```python
from build123d import *

# Parameters (mm, degrees)
CROQUIS1_R              = 0.8
CROQUIS1_R_2            = 0.5
CROQUIS1_W              = 22.5
CROQUIS1_H              = 12
SALIENTE_EXTRUIR1_DEPTH = 8
CROQUIS2_R              = 10
CORTAR_EXTRUIR1_DEPTH   = 104.387620149


with BuildPart() as part:
    # Croquis1 → Saliente-Extruir1 (new body)
    with BuildSketch(Plane.XY):
        with BuildLine():
            Line((1.5625, 24.951124098), (81.25, 19.960899278))
            ThreePointArc((81.25, 19.960899278), (100, 0), (81.25, -19.960899278))
            Line((81.25, -19.960899278), (1.5625, -24.951124098))
            ThreePointArc((1.5625, -24.951124098), (-25, 0), (1.5625, 24.951124098))
        make_face()
        Circle(CROQUIS1_R, mode=Mode.SUBTRACT)
        with Locations((66.375, 0)):
            Circle(CROQUIS1_R_2, mode=Mode.SUBTRACT)
        with Locations((93.625, 0)):
            Circle(CROQUIS1_R_2, mode=Mode.SUBTRACT)
        with Locations((7.5, 0)):
            Circle(CROQUIS1_R, mode=Mode.SUBTRACT)
        with Locations((0, -7.5)):
            Circle(CROQUIS1_R, mode=Mode.SUBTRACT)
        with Locations((-7.5, 0)):
            Circle(CROQUIS1_R, mode=Mode.SUBTRACT)
        with Locations((0, 7.5)):
            Circle(CROQUIS1_R, mode=Mode.SUBTRACT)
        with Locations((80, 0)):
            Rectangle(CROQUIS1_W, CROQUIS1_H, mode=Mode.SUBTRACT)
    extrude(amount=-SALIENTE_EXTRUIR1_DEPTH)

    # Croquis2 → Cortar-Extruir1 (cut, through all)
    with BuildSketch(Plane.XY):
        Circle(CROQUIS2_R)
    extrude(amount=-CORTAR_EXTRUIR1_DEPTH, mode=Mode.SUBTRACT)


solid = part.part
```
Model file for the job. Use its own axes, mm. A direction names the side the tool comes from. Round coordinates to 2 decimals unless told otherwise and drop trailing zeros. Write each loop counter-clockwise with the first axis right and the second up, starting at its lowest first coordinate (ties: lowest second). Pieces come first, ordered by that corner, then holes. Notation, with made-up numbers: (51.5, 60.25) -> (69.5, 60.25) arc R25 ccw to (69.5, 84.25) -> close; hole circle Ø4 at (-8.75, 86). An arc over 180 degrees is marked (long way). Answer as CSV lines item,"result".
1. Slice it at B-B, the plane z = -6.5. State how many separate pieces and enclosed holes the cut face has, plus the area to 3 significant figures.
Resolved:
separate pieces,"1"
enclosed holes,"4"
area,"4,630 mm²"
2. Pin check, flat tips, straight feed: pin 1 Ø4 at (x, z) = (76, -6) entering from +Y; pin 2 Ø2.5 at (x, z) = (84, -3.5) entering from -Y; pin 3 Ø1.5 at (x, z) = (46.5, -3) entering from -Y. Stop position of each tip, or through.
Resolved:
pin 1,"y = 20.41"
pin 2,"y = -19.81"
pin 3,"y = -22.18"
3. Slice it at A-A, the plane x = 0. List the corners of the cut face in (y, z), plus the area to 3 significant figures.
Resolved:
outline,"(-25, -8) -> (-10, -8) -> (-10, 0) -> (-25, 0) -> close; (10, -8) -> (25, -8) -> (25, 0) -> (10, 0) -> close"
area,"240 mm²"
4. Mould opens along Y. For faces 1 (the face through (40.85, 22.49, -3.94)), 2 (the face through (100, 0, -4)), 3 (the face through (91.25, 0, -4)) say: +Y half, -Y half, draft (parallel to the pull), parting line (faces both ways), or undercut.
Resolved:
face 1,"+Y half"
face 2,"parting line"
face 3,"undercut"
5. Slice it at C-C, the plane y = 7.5. List the corners of the cut face in (x, z), plus the area to 3 significant figures.
Resolved:
outline,"(-23.85, -8) -> (-6.61, -8) -> (-6.61, 0) -> (-23.85, 0) -> close; (6.61, -8) -> (98.54, -8) -> (98.54, 0) -> (6.61, 0) -> close"
area,"873 mm²"
6. Slice it at D-D, the plane y = -3. List the corners of the cut face in (x, z), plus the area to 3 significant figures.
Resolved:
outline,"(-24.82, -8) -> (-9.54, -8) -> (-9.54, 0) -> (-24.82, 0) -> close; (9.54, -8) -> (68.75, -8) -> (68.75, 0) -> (9.54, 0) -> close; (91.25, -8) -> (99.77, -8) -> (99.77, 0) -> (91.25, 0) -> close"
area,"664 mm²"
7. Drill centre lines: line 1 (Y direction, x = 0, z = -3.5); line 2 (X direction, y = -1, z = -4.5); line 3 (X direction, y = -5, z = -6.5). Where is each one in solid material? Low to high.
Resolved:
line 1,"-25 to -10, 10 to 25"
line 2,"-24.98 to -9.95, 9.95 to 68.75, 91.25 to 99.97"
line 3,"-24.49 to -8.66, 8.66 to 68.75, 91.25 to 99.36"
8. Tool access for faces 4 (the face through (38, 0, -8)), 5 (the face through (80, 6, -4)): list every direction of +Z, -Z, +X, -X, +Y, -Y with a clear straight run to the whole face (end or side of a thin tool).
Resolved:
face 4,"-Z, +X, -X, +Y, -Y"
face 5,"+Z, -Z"
